```python
from build123d import *

# Parameters (mm, degrees)
SKETCH1_W           = 30.15
SKETCH1_H           = 12.15
BOSS_EXTRUDE1_DEPTH = 2
SKETCH2_W           = 30.15
SKETCH2_H           = 12.15
SKETCH2_W_2         = 29.15
SKETCH2_H_2         = 11.15
BOSS_EXTRUDE2_DEPTH = 1
CUT_EXTRUDE1_DEPTH  = 2
SKETCH4_W           = 0.5
SKETCH4_H           = 3
CUT_EXTRUDE2_DEPTH  = 1


with BuildPart() as part:
    # Sketch1 → Boss-Extrude1 (new body)
    with BuildSketch(Plane.XY):
        Rectangle(SKETCH1_W, SKETCH1_H)
    extrude(amount=BOSS_EXTRUDE1_DEPTH)

    # Sketch2 → Boss-Extrude2 (add)
    with BuildSketch(Plane.XY.offset(2)):
        Rectangle(SKETCH2_W, SKETCH2_H)
        Rectangle(SKETCH2_W_2, SKETCH2_H_2, mode=Mode.SUBTRACT)
    extrude(amount=BOSS_EXTRUDE2_DEPTH)

    # Sketch3 → Cut-Extrude1 (cut)
    with BuildSketch(Plane(origin=(0, 0, 0), x_dir=(-1, 0, 0), z_dir=(0, 0, -1))):
        with BuildLine():
            Line((-1, -3), (-1, 3))
            ThreePointArc((-1, 3), (0, 4), (1, 3))
            Line((1, 3), (1, -3))
            ThreePointArc((1, -3), (0, -4), (-1, -3))
        make_face()
        with BuildLine():
            Line((-6, -3), (-6, 3))
            ThreePointArc((-6, 3), (-5, 4), (-4, 3))
            Line((-4, 3), (-4, -3))
            ThreePointArc((-4, -3), (-5, -4), (-6, -3))
        make_face()
        with BuildLine():
            Line((-11, -3), (-11, 3))
            ThreePointArc((-11, 3), (-10, 4), (-9, 3))
            Line((-9, 3), (-9, -3))
            ThreePointArc((-9, -3), (-10, -4), (-11, -3))
        make_face()
        with BuildLine():
            Line((4, -3), (4, 3))
            ThreePointArc((4, 3), (5, 4), (6, 3))
            Line((6, 3), (6, -3))
            ThreePointArc((6, -3), (5, -4), (4, -3))
        make_face()
        with BuildLine():
            Line((9, -3), (9, 3))
            ThreePointArc((9, 3), (10, 4), (11, 3))
            Line((11, 3), (11, -3))
            ThreePointArc((11, -3), (10, -4), (9, -3))
        make_face()
    extrude(amount=-CUT_EXTRUDE1_DEPTH, mode=Mode.SUBTRACT)

    # Sketch4 → Cut-Extrude2 (cut)
    with BuildSketch(Plane.XY.offset(3)):
        with Locations((-14.825, 0)):
            Rectangle(SKETCH4_W, SKETCH4_H)
        with Locations((14.825, 0)):
            Rectangle(SKETCH4_W, SKETCH4_H)
    extrude(amount=-CUT_EXTRUDE2_DEPTH, mode=Mode.SUBTRACT)


solid = part.part
```
Here's how the part is built. I have some questions about the finished solid (model axes, mm). A direction names the side the tool comes from. Round coordinates to 2 decimals unless told otherwise and drop trailing zeros. Order: outer loops, then holes, each group sorted by start corner. A loop starts at its lowest first (then second) coordinate and runs counter-clockwise, first axis right, second up. Notation, with made-up numbers: (59, 4) -> (82, 4) arc R10 ccw to (82, 12) -> close; hole circle Ø8 at (29, 43). An arc over 180 degrees is marked (long way). Use a Markdown table: item, result. Add a question column.
(1) Suppose I cut it at B-B, the plane x = 5. Please give me the cut outline in (y, z) (3 decimals), and give its area (3 significant figures).
(2) For faces 4 (the face through (-4.5, 5.8, 3)), 5 (the face through (-1, 0, 1)), 6 (the face through (14.575, -3.6, 2.5)), which set-ups out of +Z, -Z, +X, -X, +Y, -Y let a thin tool reach every point of the face, with its end or its side?
(3) If we mould it in two halves opening along X, with no side actions, what happens to faces 1 (the face through (5, -4, 1)), 2 (the face through (15.075, 0, 1)), 3 (the face through (0, -6.075, 1))? For each: released by +X, released by -X, zero draft, split by the parting line, or undercut.
(4) Suppose I cut it at C-C, the plane z = 1.2. Please give me the cut outline in (x, y) (3 decimals), and give its area (3 significant figures).
(5) Suppose I cut it at A-A, the plane y = 0.5. Please give me the cut outline in (x, z) (3 decimals), and give its area (3 significant figures).
(6) Suppose I cut it at D-D, the plane x = -13. Please give me the cut outline in (y, z) (3 decimals).
(7) I need wall thicknesses on line 1 along X through (y, z) = (0, 0.8) (3 decimals); line 2 along Y through (x, z) = (0, 2.3) (3 decimals); line 3 along X through (y, z) = (5.25, 2.1) (3 decimals). Which ranges of each line are inside material? Lowest first, please.
Verdict:
| question | item | result |
|---|---|---|
| 1 | outline | (-6.075, 0) -> (-4, 0) -> (-4, 2) -> (-5.575, 2) -> (-5.575, 3) -> (-6.075, 3) -> close; (4, 0) -> (6.075, 0) -> (6.075, 3) -> (5.575, 3) -> (5.575, 2) -> (4, 2) -> close |
| 1 | area | 9.30 mm2 |
| 2 | face 4 | +Z, +X, -X, +Y, -Y |
| 2 | face 5 | +Z, -Z |
| 2 | face 6 | +Z |
| 3 | face 1 | undercut |
| 3 | face 2 | released by +X |
| 3 | face 3 | zero draft |
| 4 | outline | (-15.075, -6.075) -> (15.075, -6.075) -> (15.075, 6.075) -> (-15.075, 6.075) -> close; hole (-11, -3) arc R1 ccw to (-9, -3) -> (-9, 3) arc R1 ccw to (-11, 3) -> close; hole (-6, -3) arc R1 ccw to (-4, -3) -> (-4, 3) arc R1 ccw to (-6, 3) -> close; hole (-1, -3) arc R1 ccw to (1, -3) -> (1, 3) arc R1 ccw to (-1, 3) -> close; hole (4, -3) arc R1 ccw to (6, -3) -> (6, 3) arc R1 ccw to (4, 3) -> close; hole (9, -3) arc R1 ccw to (11, -3) -> (11, 3) arc R1 ccw to (9, 3) -> close |
| 4 | area | 291 mm2 |
| 5 | outline | (-15.075, 0) -> (-11, 0) -> (-11, 2) -> (-15.075, 2) -> close; (-9, 0) -> (-6, 0) -> (-6, 2) -> (-9, 2) -> close; (-4, 0) -> (-1, 0) -> (-1, 2) -> (-4, 2) -> close; (1, 0) -> (4, 0) -> (4, 2) -> (1, 2) -> close; (6, 0) -> (9, 0) -> (9, 2) -> (6, 2) -> close; (11, 0) -> (15.075, 0) -> (15.075, 2) -> (11, 2) -> close |
| 5 | area | 40.3 mm2 |
| 6 | outline | (-6.075, 0) -> (6.075, 0) -> (6.075, 3) -> (5.575, 3) -> (5.575, 2) -> (-5.575, 2) -> (-5.575, 3) -> (-6.075, 3) -> close |
| 7 | line 1 | -15.075 to -11, -9 to -6, -4 to -1, 1 to 4, 6 to 9, 11 to 15.075 |
| 7 | line 2 | -6.075 to -5.575, 5.575 to 6.075 |
| 7 | line 3 | -15.075 to -14.575, 14.575 to 15.075 |
